Verification items for the finished model (mm, model axes). Round coordinates to 2 decimals unless told otherwise and drop trailing zeros. Write each loop counter-clockwise with the first axis right and the second up, starting at its lowest first coordinate (ties: lowest second). Pieces come first, ordered by that corner, then holes. Notation, with made-up numbers: M -10,40 L 32,40 A29 cw 32,71 Z; hole C 76.5,76.5 d4. An arc over 180 degrees is marked long. Answer in a Markdown table with one row per item. Add a question column.
1. Go/stop test with flat-tipped pins: pin 1 Ø3 at (x, z) = (-103, 0.5) entering from -Y (3 decimals); pin 2 Ø2.5 at (x, y) = (-104, 0.5) entering from -Z; pin 3 Ø2 at (x, y) = (-63.5, 1) entering from -Z. Record where each tip stops, or that it passes through.
2. Material ranges on probe 1 along X at (y, z) = (3.25, 4.5); probe 2 along X at (y, z) = (-0.5, 0.5); probe 3 along Y at (x, z) = (-6, 0.5), recorded low to high.
3. Sectioned sample at A-A on x = -15. Record the cut outline in (y, z).
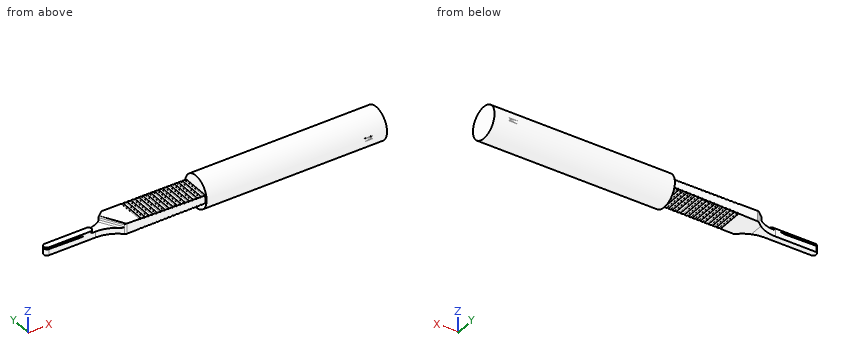
```python
from build123d import *

# Parameters (mm, degrees)
BOSS_EXTRU_1_DEPTH           = 2
CONG_2_R                     = 1
ENL_V_MAT_EXTRU_1_DEPTH      = 1.77
CONG_1_R                     = 0.5
ENL_V_MAT_EXTRU_2_DEPTH      = 120.16794871273063
ENL_V_MAT_EXTRU_2_DEPTH_BACK = 120.16794871273063
ESQUISSE4_OUTSIDE_W          = 152.128
ESQUISSE4_OUTSIDE_H          = 31.128000000000004
ENL_V_MAT_EXTRU_3_DEPTH      = 120.16794871273063
R_P_TITION_START             = -5.329109723
R_P_TITION_LIN_AIRE1_DEPTH   = 10.672345711
ENL_V_MAT_EXTRU_5_DEPTH      = 0.19
BOSS_EXTRU_2_DEPTH           = 6
BOSS_EXTRU_2_DEPTH_BACK      = 61.78718
ESQUISSE9_R                  = 6


# Read off the part's stored shape, not the designer's step: Répétition linéaire1
with BuildPart() as part:
    # Esquisse1 → Boss.-Extru.1 (new, symmetric)
    with BuildSketch(Plane.XY):
        with BuildLine():
            Line((-94, 5.000654392557492), (-0.06380606653039397, 5.999660722563728))
            ThreePointArc((-0.06380606653039397, 5.999660722563728), (5.999999960724106, -0.0006865206484478), (-0.06517902850728707, -5.9996459640751185))
            Line((-0.06517902850728707, -5.9996459640751185), (-91.5, -5.0063152178369394))
            ThreePointArc((-91.5, -5.0063152178369394), (-95.49287183308192, -2.181722820314924), (-100.28117960378982, -1.1850000000000003))
            Line((-100.28117960378982, -1.1850000000000003), (-117.815, -1.185))
            ThreePointArc((-117.815, -1.185), (-119, 1.5e-16), (-117.815, 1.185))
            Line((-117.815, 1.185), (-102.77590376986532, 1.1850000000000003))
            ThreePointArc((-102.77590376986532, 1.1850000000000003), (-97.99114396864803, 2.1801795269229824), (-94, 5.000654392557492))
        make_face()
    extrude(amount=BOSS_EXTRU_1_DEPTH, both=True)

    # Congé2
    cong_2_edges = [part.edges().sort_by_distance(p)[0] for p in [
        (-91.5, -5.006315217836939, 0),
        (-94, 5.000654392557493, 0),
    ]]
    fillet(cong_2_edges, radius=CONG_2_R)

    # Esquisse3 → Enlèv. mat.-Extru.1 (cut)
    with BuildSketch(Plane.XY.offset(2)):
        with BuildLine():
            Line((-97.36861768988254, 4.964829326045353), (-91.6124802044987, -5.005093253991168))
            Line((-91.6124802044987, -5.005093253991168), (-102.18500000000003, -5.00509325399117))
            Line((-102.18500000000003, -5.00509325399117), (-102.18500000000003, -1.185))
            ThreePointArc((-102.18500000000003, -1.185), (-101.00000000000003, 0), (-102.18500000000003, 1.185))
            Line((-102.18500000000003, 1.185), (-102.18500000000003, 4.964829326045353))
            Line((-102.18500000000003, 4.964829326045353), (-97.36861768988254, 4.964829326045353))
        make_face()
    extrude(amount=-ENL_V_MAT_EXTRU_1_DEPTH, mode=Mode.SUBTRACT)

    # Congé1
    cong_1_edges = [part.edges().sort_by_distance(p)[0] for p in [
        (-94.03287302320349, -0.8128499177196291, 0.22999999999999998),
        (-94.03287302320348, -0.8128499177196522, 2),
    ]]
    fillet(cong_1_edges, radius=CONG_1_R)

    # Esquisse4 outside → Enlèv. mat.-Extru.2 (cut, two sides: drawn at the far end of the back side and taken through both)
    with BuildSketch(Plane(origin=(0, 0, 0), x_dir=(1, 0, 0), z_dir=(0, 1, 0)).offset(-ENL_V_MAT_EXTRU_2_DEPTH_BACK)):
        with Locations((-56.5, 0)):
            Rectangle(ESQUISSE4_OUTSIDE_W, ESQUISSE4_OUTSIDE_H)
        Polygon((-119.00000000000001, -1.000000000000003), (-99, -1.000000000000003), (-95.8708882867572, -2), (6, -0.5), (6, 0.5), (-95.8708882867572, 2), (-119.00000000000001, 2), align=None, mode=Mode.SUBTRACT)
    extrude(amount=ENL_V_MAT_EXTRU_2_DEPTH + ENL_V_MAT_EXTRU_2_DEPTH_BACK, mode=Mode.SUBTRACT)

    # Esquisse5 → Enlèv. mat.-Extru.3 (cut, symmetric)
    with BuildSketch(Plane(origin=(0, 0, 0), x_dir=(1, 0, 0), z_dir=(0, 1, 0))):
        with BuildLine():
            Line((-86.38322192363898, 1.8602986605494507), (-85.78322192363899, 1.8514639481489208))
            ThreePointArc((-85.78322192363899, 1.8514639481489208), (-86.08616650857984, 1.6559029819751625), (-86.38322192363898, 1.8602986605494507))
        make_face()
    enl_v_mat_extru_3 = extrude(amount=ENL_V_MAT_EXTRU_3_DEPTH, both=True, mode=Mode.SUBTRACT)

    # Répétition linéaire1 outline → Répétition linéaire1 (cut)
    with BuildSketch(Plane(origin=(0, 0, 0), x_dir=(1, 0, 0), z_dir=(0, 1, 0)).offset(R_P_TITION_START)):
        with BuildLine():
            Line((-84.283469298, 1.82938081), (-84.883469298, 1.838215522))
            ThreePointArc((-84.883469298, 1.838215522), (-84.586413883, 1.633819843), (-84.283469298, 1.82938081))
        make_face()
        with BuildLine():
            Line((-61.787179907, 1.498133732), (-62.387179907, 1.506968444))
            ThreePointArc((-62.387179907, 1.506968444), (-62.090124492, 1.302572765), (-61.787179907, 1.498133732))
        make_face()
        with BuildLine():
            Line((-63.286932533, 1.52021687), (-63.886932533, 1.529051582))
            ThreePointArc((-63.886932533, 1.529051582), (-63.589877118, 1.324655904), (-63.286932533, 1.52021687))
        make_face()
        with BuildLine():
            Line((-64.786685159, 1.542300009), (-65.386685159, 1.551134721))
            ThreePointArc((-65.386685159, 1.551134721), (-65.089629744, 1.346739042), (-64.786685159, 1.542300009))
        make_face()
        with BuildLine():
            Line((-66.286437785, 1.564383147), (-66.886437785, 1.57321786))
            ThreePointArc((-66.886437785, 1.57321786), (-66.58938237, 1.368822181), (-66.286437785, 1.564383147))
        make_face()
        with BuildLine():
            Line((-67.786190411, 1.586466286), (-68.386190411, 1.595300998))
            ThreePointArc((-68.386190411, 1.595300998), (-68.089134996, 1.39090532), (-67.786190411, 1.586466286))
        make_face()
        with BuildLine():
            Line((-69.285943037, 1.608549424), (-69.885943037, 1.617384137))
            ThreePointArc((-69.885943037, 1.617384137), (-69.588887622, 1.412988458), (-69.285943037, 1.608549424))
        make_face()
        with BuildLine():
            Line((-70.785695663, 1.630632563), (-71.385695663, 1.639467275))
            ThreePointArc((-71.385695663, 1.639467275), (-71.088640248, 1.435071597), (-70.785695663, 1.630632563))
        make_face()
        with BuildLine():
            Line((-72.285448289, 1.652715701), (-72.885448289, 1.661550414))
            ThreePointArc((-72.885448289, 1.661550414), (-72.588392874, 1.457154735), (-72.285448289, 1.652715701))
        make_face()
        with BuildLine():
            Line((-73.785200915, 1.67479884), (-74.385200915, 1.683633552))
            ThreePointArc((-74.385200915, 1.683633552), (-74.0881455, 1.479237874), (-73.785200915, 1.67479884))
        make_face()
        with BuildLine():
            Line((-75.284953541, 1.696881978), (-75.884953541, 1.705716691))
            ThreePointArc((-75.884953541, 1.705716691), (-75.587898126, 1.501321012), (-75.284953541, 1.696881978))
        make_face()
        with BuildLine():
            Line((-76.784706168, 1.718965117), (-77.384706168, 1.727799829))
            ThreePointArc((-77.384706168, 1.727799829), (-77.087650753, 1.523404151), (-76.784706168, 1.718965117))
        make_face()
        with BuildLine():
            Line((-78.284458794, 1.741048255), (-78.884458794, 1.749882968))
            ThreePointArc((-78.884458794, 1.749882968), (-78.587403379, 1.545487289), (-78.284458794, 1.741048255))
        make_face()
        with BuildLine():
            Line((-79.78421142, 1.763131394), (-80.38421142, 1.771966106))
            ThreePointArc((-80.38421142, 1.771966106), (-80.087156005, 1.567570428), (-79.78421142, 1.763131394))
        make_face()
        with BuildLine():
            Line((-81.283964046, 1.785214533), (-81.883964046, 1.794049245))
            ThreePointArc((-81.883964046, 1.794049245), (-81.586908631, 1.589653566), (-81.283964046, 1.785214533))
        make_face()
        with BuildLine():
            Line((-82.783716672, 1.807297671), (-83.383716672, 1.816132383))
            ThreePointArc((-83.383716672, 1.816132383), (-83.086661257, 1.611736705), (-82.783716672, 1.807297671))
        make_face()
    r_p_tition_lin_aire1 = extrude(amount=R_P_TITION_LIN_AIRE1_DEPTH, mode=Mode.SUBTRACT)

    # Symétrie1: Enlèv. mat.-Extru.3, Répétition linéaire1 across plane
    add(enl_v_mat_extru_3.mirror(Plane.XY), mode=Mode.SUBTRACT)
    add(r_p_tition_lin_aire1.mirror(Plane.XY), mode=Mode.SUBTRACT)

    # Esquisse8 → Enlèv. mat.-Extru.5 (cut, symmetric)
    with BuildSketch(Plane(origin=(-0.02696303982545021, 0, -1.5447115170486774), x_dir=(0.9998476951563913, 0, -0.01745240643728355), z_dir=(0.01745240643728355, 0, 0.9998476951563913))):
        with BuildLine():
            Line((-117.81450861128754, -0.6849999999999998), (-107.93700761048673, -0.6849999999999998))
            ThreePointArc((-107.93700761048673, -0.6849999999999998), (-106.35586878040255, -0.8107911709342499), (-104.81450861128754, -1.1849999999999998))
            Line((-104.81450861128754, -1.1849999999999998), (-104.81450861128754, -1.6849999999999998))
            Line((-104.81450861128754, -1.6849999999999998), (-117.81450861128754, -1.6849999999999998))
            ThreePointArc((-117.81450861128754, -1.6849999999999998), (-119.49950861128754, 2.1e-16), (-117.81450861128754, 1.685))
            Line((-117.81450861128754, 1.685), (-104.81450861128754, 1.6850000000000016))
            Line((-104.81450861128754, 1.6850000000000016), (-104.81450861128754, 1.185))
            ThreePointArc((-104.81450861128754, 1.185), (-106.35586878040255, 0.8107911709342517), (-107.93700761048673, 0.6850000000000016))
            Line((-107.93700761048673, 0.6850000000000016), (-117.81450861128754, 0.6849999999999999))
            ThreePointArc((-117.81450861128754, 0.6849999999999999), (-118.49950861128754, 8e-17), (-117.81450861128754, -0.6849999999999998))
        make_face()
    extrude(amount=ENL_V_MAT_EXTRU_5_DEPTH, both=True, mode=Mode.SUBTRACT)

    # Esquisse9 → Boss.-Extru.2 (add, two sides: drawn at the far end of the back side and taken through both)
    with BuildSketch(Plane(origin=(0, 0, 0), x_dir=(0, 0, -1), z_dir=(1, 0, 0)).offset(-BOSS_EXTRU_2_DEPTH_BACK)):
        Circle(ESQUISSE9_R)
    extrude(amount=BOSS_EXTRU_2_DEPTH + BOSS_EXTRU_2_DEPTH_BACK)


solid = part.part
```
Geometry check:
| question | item | result |
|---|---|---|
| 1 | pin 1 | stops at y = -1.185 |
| 1 | pin 2 | stops at z = -2 |
| 1 | pin 3 | stops at z = -1.54 |
| 2 | probe 1 | x = -61.79 to 6 |
| 2 | probe 2 | x = -118.29 to -101.11, -94.28 to 6 |
| 2 | probe 3 | y = -5.98 to 5.98 |
| 3 | outline | C 0,0 d12 |
